Build history of the part. All positions in model axes, mm. Give positions to 0.01 mm unless a question says otherwise; leave off trailing zeros. Write each loop counter-clockwise with the first axis right and the second up, starting at its lowest first coordinate (ties: lowest second). Pieces come first, ordered by that corner, then holes. Notation, with made-up numbers: (55, -33) -> (95, -33) arc R20 ccw to (95, 0) -> close; hole circle Ø5 at (-5, 88.5). An arc over 180 degrees is marked (long way). Put each result on its own line as item: value.
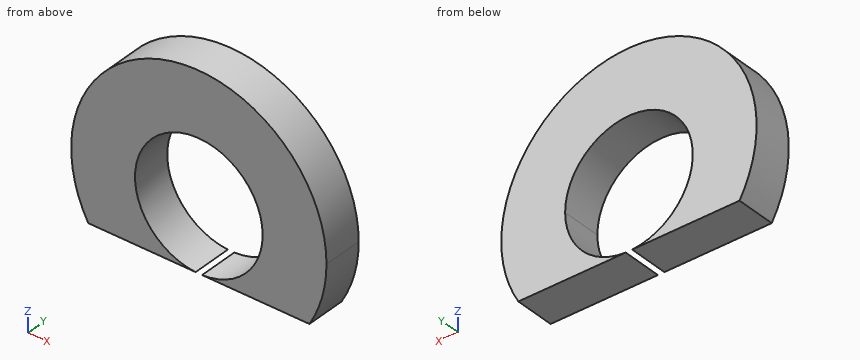
from build123d import *

# Parameters (mm, degrees)
F1_DEPTH = 2.5


# Not quite as in the source:
# - a feature names something its author has since deleted; it is built from what else it names


with BuildPart() as f1:
    # F0 (on Front) → F1 (new body)
    with BuildSketch(Plane.XZ):
        with BuildLine():
            ThreePointArc((-0.2018715048, -3.3093462615), (-2.7561308007, 3.5844774855), (4, 0.6855564776))
            ThreePointArc((4, 0.6855564776), (2.8989210078, -2.070574323), (0.2018715048, -3.3093462615))
            Line((0.2018715048, -3.3093462615), (4.4766898602, -3.3093462615))
            ThreePointArc((4.4766898602, -3.3093462615), (5.6062527218, -1.4521830807), (6, 0.6855564776))
            ThreePointArc((6, 0.6855564776), (-2.1377395584, 6.2918091994), (-4.4766898602, -3.3093462615))
            Line((-4.4766898602, -3.3093462615), (-0.2018715048, -3.3093462615))
        make_face()
        with BuildLine():
            Line((-6.9311436361, -3.3093462615), (-4.4766898602, -3.3093462615))
            ThreePointArc((-4.4766898602, -3.3093462615), (-2.1377395584, 6.2918091994), (6, 0.6855564776))
            ThreePointArc((6, 0.6855564776), (5.6062527218, -1.4521830807), (4.4766898602, -3.3093462615))
            Line((4.4766898602, -3.3093462615), (6.9311436361, -3.3093462615))
            ThreePointArc((6.9311436361, -3.3093462615), (7.7281676059, -1.3821537186), (8, 0.6855564776))
            ThreePointArc((8, 0.6855564776), (-2.0677101962, 8.4137240835), (-6.9311436361, -3.3093462615))
        make_face()
    extrude(amount=F1_DEPTH)


solid = f1.part
1) Slice it at A-A (z = 2.5). Write the cut outline in (x, y).
Filled sheet:
outline: (-7.79, -2.5) -> (-3.56, -2.5) -> (-3.56, 0) -> (-7.79, 0) -> close; (3.56, -2.5) -> (7.79, -2.5) -> (7.79, 0) -> (3.56, 0) -> close
2) Slice it at B-B (x = -2). Write the cut outline in (y, z), plus the area to 3 significant figures.
Filled sheet:
outline: (-2.5, -3.31) -> (0, -3.31) -> (0, -2.78) -> (-2.5, -2.78) -> close; (-2.5, 4.15) -> (0, 4.15) -> (0, 8.43) -> (-2.5, 8.43) -> close
area: 12.0 mm2
3) Slice it at D-D (x = 0). Write the cut outline in (y, z), plus the area to 4 significant figures.
Filled sheet:
outline: (-2.5, 4.69) -> (0, 4.69) -> (0, 8.69) -> (-2.5, 8.69) -> close
area: 10.00 mm2
4) Wall check: L1, parallel to Z at x = 0, y = -1.9; L2, parallel to X at y = -0.2, z = 3.5; L3, parallel to X at y = -2.2, z = 3.75. Give the ranges that are in metal, low to high.
Filled sheet:
L1: 4.69 to 8.69
L2: -7.49 to -2.84, 2.84 to 7.49
L3: -7.39 to -2.57, 2.57 to 7.39
5) Slice it at C-C (y = -0.2). Write the cut outline in (x, z).
Filled sheet:
outline: (-6.93, -3.31) -> (-0.2, -3.31) arc R4 cw (long way) to (0.2, -3.31) -> (6.93, -3.31) arc R8 ccw (long way) to start
